Check sheet for the drawn part. Datum: minimum x, y, z corner. Units: mm. A direction names the side the tool comes from. Round coordinates to 2 decimals unless told otherwise and drop trailing zeros. Write each loop counter-clockwise with the first axis right and the second up, starting at its lowest first coordinate (ties: lowest second). Pieces come first, ordered by that corner, then holes. Notation, with made-up numbers: M 67,15 L 83,15 A19 ccw 83,32 Z; hole C -15,62 d8. An arc over 180 degrees is marked long. Use a Markdown table: item, result.
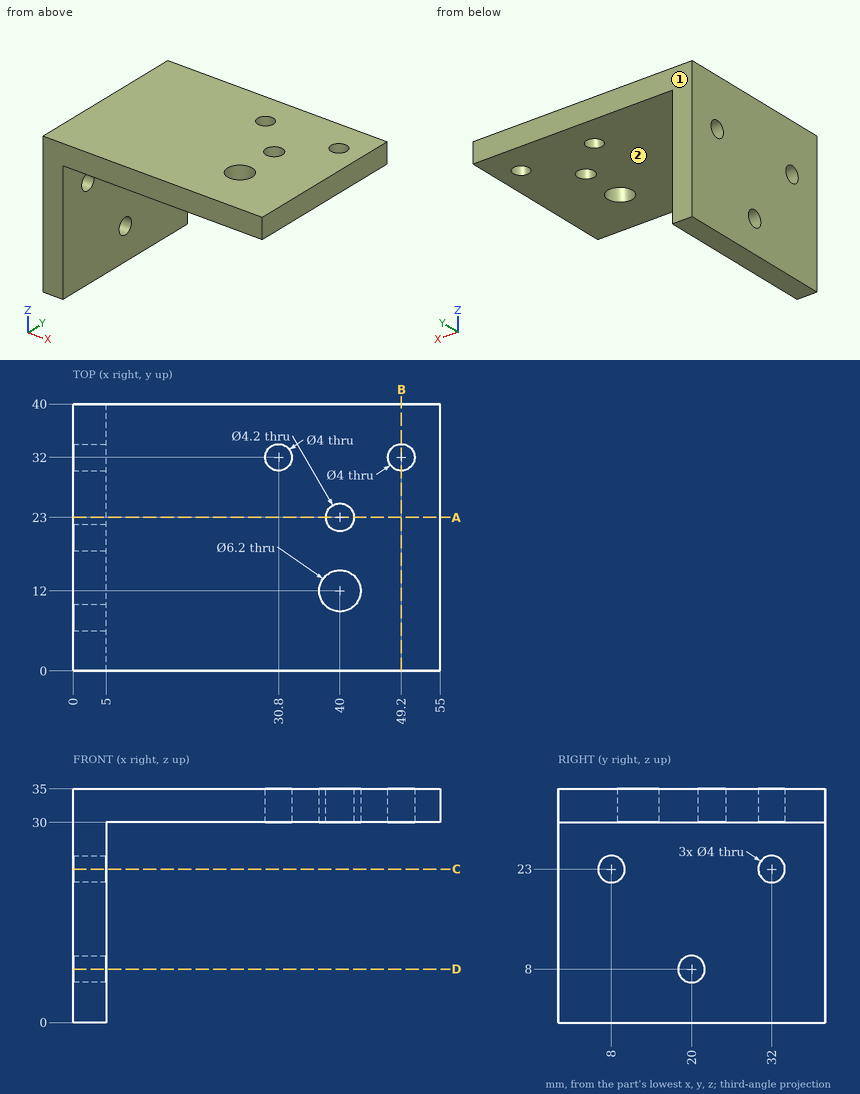
Item 1: Cross-section at C-C, the plane z = 23. Record the cut outline in (x, y).
Outcome:
| item | result |
|---|---|
| outline | M 0,0 L 5,0 L 5,6 L 0,6 Z; M 0,10 L 5,10 L 5,30 L 0,30 Z; M 0,34 L 5,34 L 5,40 L 0,40 Z |
Item 2: Access from +Z, -Z, +X, -X, +Y, -Y to the whole of each face (thin tool, end or side, straight path). Record for the marked faces 1 and 2.
Outcome:
| item | result |
|---|---|
| face 1 | +Z, -Z, +X, -X, +Y |
| face 2 | -Z, +X, +Y, -Y |
Item 3: Cross-section at D-D, the plane z = 8. Record the cut outline in (x, y).
Outcome:
| item | result |
|---|---|
| outline | M 0,0 L 5,0 L 5,18 L 0,18 Z; M 0,22 L 5,22 L 5,40 L 0,40 Z |
Item 4: Material ranges on line 1 along Y through (x, z) = (49, 31); line 2 along Y through (x, z) = (40, 33); line 3 along X through (y, z) = (30, 17), recorded low to high. Write a range as from..to.
Outcome:
| item | result |
|---|---|
| line 1 | y = 0..30.01, 33.99..40 |
| line 2 | y = 0..8.9, 15.1..20.9, 25.1..40 |
| line 3 | x = 0..5 |
Item 5: Go/stop test with flat-tipped pins: pin 1 (1 mm diameter, centred on x = 44, y = 18.5, fed in from -Z); pin 2 (1 mm diameter, centred on y = 24, z = 16.5, fed in from +X); pin 3 (5.5 mm diameter, centred on x = 40, y = 23, fed in from +Z). Record where each tip stops, or that it passes through.
Outcome:
| item | result |
|---|---|
| pin 1 | stops at z = 30 |
| pin 2 | stops at x = 5 |
| pin 3 | stops at z = 35 |
Item 6: Cross-section at B-B, the plane x = 49.2. Record the cut outline in (y, z).
Outcome:
| item | result |
|---|---|
| outline | M 0,30 L 30,30 L 30,35 L 0,35 Z; M 34,30 L 40,30 L 40,35 L 34,35 Z |
Item 7: Cross-section at A-A, the plane y = 23. Record the cut outline in (x, z).
Outcome:
| item | result |
|---|---|
| outline | M 0,0 L 5,0 L 5,30 L 37.9,30 L 37.9,35 L 0,35 Z; M 42.1,30 L 55,30 L 55,35 L 42.1,35 Z |
